Input: part model. Units: mm. Frame: model coordinates. A direction names the side the tool comes from. Coordinates: 2 decimals unless noted, no trailing zeros. Write each loop counter-clockwise with the first axis right and the second up, starting at its lowest first coordinate (ties: lowest second). Pieces come first, ordered by that corner, then holes. Notation, with made-up numbers: M 46,68 L 85,68 A22 cw 85,106 Z; hole C -21.5,6 d5. An arc over 180 degrees is marked long. Use one line per item in the form item = value.
from build123d import *

# Parameters (mm, degrees)
SKETCH_1_W          = 12
SKETCH_1_H          = 12
EXTRUDE_1_DEPTH     = 110
SKETCH_2_W          = 7
SKETCH_2_H          = 7
CUT_EXTRUDE_1_DEPTH = 111.326787318
SKETCH_3_R          = 1.6
SKETCH_3_R_2        = 1.55
CUT_EXTRUDE_2_DEPTH = 111.815161418


with BuildPart() as part:
    # 草图1 → 凸台-拉伸1 (new body)
    with BuildSketch(Plane.XY):
        Rectangle(SKETCH_1_W, SKETCH_1_H)
    extrude(amount=EXTRUDE_1_DEPTH)

    # 草图2 → 切除-拉伸1 (cut, through all)
    with BuildSketch(Plane.XY.offset(110)):
        Rectangle(SKETCH_2_W, SKETCH_2_H)
    extrude(amount=-CUT_EXTRUDE_1_DEPTH, mode=Mode.SUBTRACT)

    # 草图3 → 切除-拉伸2 (cut, through all)
    with BuildSketch(Plane.XZ.offset(6)):
        with Locations(Location((0, 7, 0), (0, 0, 270))):
            Circle(SKETCH_3_R)
        with Locations(Location((0, 17, 0), (0, 0, 270))):
            Circle(SKETCH_3_R)
        with Locations(Location((0, 102.5, 0), (0, 0, 270))):
            Circle(SKETCH_3_R_2)
    extrude(amount=-CUT_EXTRUDE_2_DEPTH, mode=Mode.SUBTRACT)


solid = part.part
(1) Line query: probe 1 along X at (y, z) = (2, 13); probe 2 along X at (y, z) = (4.6, 7); probe 3 along Z at (x, y) = (-0.5, 4). Output: solid intervals per line, ascending.
Computed:
probe_1 = -6 to -3.5, 3.5 to 6
probe_2 = -6 to -1.6, 1.6 to 6
probe_3 = 0 to 5.48, 8.52 to 15.48, 18.52 to 101.03, 103.97 to 110
(2) Pull-direction query (X, two-part tool) for faces 1 (the flat face through (-6, 0, 54)), 2 (the flat face through (6, 0, 54)), 3 (the cylindrical face through (-0.94, 4.73, 103.73)), 4 (the flat face through (0, 6, 54)); classes: pulls with the +X half, pulls with the -X half, needs draft (parallel to the pull), parting line crosses it, or undercut.
Computed:
face_1 = pulls with the -X half
face_2 = pulls with the +X half
face_3 = undercut
face_4 = needs draft
(3) Section query B-B on x = 0. State how many separate pieces and enclosed holes the cut face has, plus the area to 4 significant figures.
Computed:
separate_pieces = 8
enclosed_holes = 0
area = 502.5 mm^2
(4) Section query C-C on z = 7. Return the cut outline in (x, y).
Computed:
outline = M -6,-6 L -1.6,-6 L -1.6,-3.5 L -3.5,-3.5 L -3.5,3.5 L -1.6,3.5 L -1.6,6 L -6,6 Z; M 1.6,-6 L 6,-6 L 6,6 L 1.6,6 L 1.6,3.5 L 3.5,3.5 L 3.5,-3.5 L 1.6,-3.5 Z
(5) Section query D-D on z = 35.5. Return the cut outline in (x, y).
Computed:
outline = M -6,-6 L 6,-6 L 6,6 L -6,6 Z; hole M -3.5,-3.5 L 3.5,-3.5 L 3.5,3.5 L -3.5,3.5 Z
(6) First-contact query: pin 1 Ø3 at (x, z) = (0, 7) entering from -Y. Flat tip, straight axial feed; report the tip coordinate or a pass-through.
Computed:
pin_1 = through
(7) Set-up query: faces 5 (the flat face through (0, 3.5, 56)), 6 (the flat face through (0, -6, 54)). Return all of +Z, -Z, +X, -X, +Y, -Y with unobstructed straight access to the full face (end or side cutting, diameter ignored); none if empty.
Computed:
face_5 = +Z, -Z
face_6 = +Z, -Z, +X, -X, -Y
(8) Section query A-A on y = -0.5. Return the cut outline in (x, z).
Computed:
outline = M -6,0 L -3.5,0 L -3.5,110 L -6,110 Z; M 3.5,0 L 6,0 L 6,110 L 3.5,110 Z
